```python
from build123d import *

# Parameters (mm, degrees)
BOSS_EXTRUDE1_DEPTH = 27.94
CIRPATTERN1_COUNT   = 17
SKETCH5_R           = 7.9375
SKETCH5_W           = 9.525
SKETCH5_H           = 11.576298251
CUT_EXTRUDE1_DEPTH  = 12.7
SKETCH5_2_R         = 7.9375
CUT_EXTRUDE2_DEPTH  = 70


with BuildPart() as part:
    # Sketch2 → Revolve1 (revolve)
    with BuildSketch(Plane(origin=(0, 0, 0), x_dir=(1, 0, 0), z_dir=(0, 1, 0))):
        Polygon((0, -14.35), (0, -58.593750066), (-19.05, -58.593750066), (-19.05, -45.893750066), (-21, -45.893750066), (-21, -35.1), (-20, -35.1), (-20, -28.1), (-18.8, -14.35), align=None)
    revolve(axis=Axis((0, 0, 14.35), (0, 0, 1)))

    # Sketch4 → Boss-Extrude1 (add)
    with BuildSketch(Plane.XY):
        with BuildLine():
            Line((-3.454490935, 18.479894274), (-3.774098097, 16.37058898))
            ThreePointArc((-3.774098097, 16.37058898), (-4.597538233, 16.158670805), (-5.40920169, 15.905361897))
            Line((-5.40920169, 15.905361897), (-6.791343324, 17.530477913))
            Line((-6.791343324, 17.530477913), (0, 0))
            Line((0, 0), (0, 18.8))
            ThreePointArc((0, 18.8), (-1.734645158, 18.719802514), (-3.454490935, 18.479894274))
        make_face()
    boss_extrude1 = extrude(amount=BOSS_EXTRUDE1_DEPTH)

    # CirPattern1: Boss-Extrude1 ×17 about axis
    cirpattern1_axis = Axis((0, 0, 0), (0, 0, 1))
    for i in range(1, CIRPATTERN1_COUNT):
        add(boss_extrude1.rotate(cirpattern1_axis, i * 360 / CIRPATTERN1_COUNT))

    # Sketch5 → Cut-Extrude1 (cut)
    with BuildSketch(Plane.XY.offset(58.593750066)):
        Circle(SKETCH5_R)
        with Locations((0, 19.470732312)):
            Rectangle(SKETCH5_W, SKETCH5_H)
    extrude(amount=-CUT_EXTRUDE1_DEPTH, mode=Mode.SUBTRACT)

    # Sketch5_2 → Cut-Extrude2 (cut)
    with BuildSketch(Plane.XY.offset(58.593750066)):
        Circle(SKETCH5_2_R)
    extrude(amount=-CUT_EXTRUDE2_DEPTH, mode=Mode.SUBTRACT)


solid = part.part
```
Check sheet for the modelled part. Datum: model origin and axes. Units: mm. A direction names the side the tool comes from. Coordinates: 2 decimals unless noted, no trailing zeros. Write each loop counter-clockwise with the first axis right and the second up, starting at its lowest first coordinate (ties: lowest second). Pieces come first, ordered by that corner, then holes. Notation, with made-up numbers: M -27.5,54.5 L -11.5,54.5 A21 ccw -11.5,83.5 Z; hole C 24.5,-7.5 d11. An arc over 180 degrees is marked long. Write item = value, one per line. Start each with the question number.
1. Tool access check on faces 1 (the flat face through (-4.762, 16, 52)), 2 (the flat face through (-14.419, 10.455, 7.075)), 3 (the flat face through (17.032, 5.206, 7.075)), 4 (the cylindrical face through (12.407, -11.327, 7.075)), 5 (the flat face through (2.917, -17.541, 7.075)). Record the directions out of +Z, -Z, +X, -X, +Y, -Y that give a thin tool (end or side, any length) a straight path to the whole face; none if there is none.
2. Thickness scan on probe 1 along Y at (x, z) = (0, 40); probe 2 along X at (y, z) = (0.5, 17.5); probe 3 along X at (y, z) = (-17, 9). Record the ranges inside material, lowest first.
3. Sectioned sample at D-D (z = 19). Record the cut outline in (x, y) (1 decimal).
4. Sectioned sample at C-C (z = 26). Record the cut outline in (x, y) (1 decimal).
5. Sectioned sample at A-A (y = 0). Record the cut outline in (x, z), then the cut area to 3 significant figures.
6. Mould release check, pull along X, two halves, no side actions. Record for faces 6 (the flat face through (-11.714, 13.378, 7.075)), 7 (the cylindrical face through (18.484, 3.431, 7.075)), 8 (the flat face through (-19, 8, 35.1)), 9 (the cylindrical face through (-14.29, -8.83, 7.07)): pulls with the +X half, pulls with the -X half, needs draft (parallel to the pull), parting line crosses it, or undercut.
7. Go/stop test with flat-tipped pins: pin 1 (0.8 mm diameter, centred on x = -5, y = 17.5, fed in from -Z); pin 2 (5 mm diameter, centred on y = 5, z = 42, fed in from -X); pin 3 (12.5 mm diameter, centred on x = 0, y = 0, fed in from +Z); pin 4 (5 mm diameter, centred on x = -9, z = 24, fed in from -Y). Record where each tip stops, or that it passes through.
The answers:
q1.face_1 = +Z, +Y
q1.face_2 = -Z, -X
q1.face_3 = -Z, +X
q1.face_4 = -Z
q1.face_5 = -Z, -Y
q2.probe_1 = -21 to -7.94, 7.94 to 21
q2.probe_2 = -19.07 to -7.92, 7.92 to 19.07
q2.probe_3 = -8.03 to -6.34, -3.68 to 0.63, 2.61 to 6.77
q3.outline = C 0,0 d38.4; hole C 0,0 d15.9
q4.outline = C 0,0 d39.6; hole C 0,0 d15.9
q5.outline = M -21,35.1 L -20,35.1 L -20,28.1 L -18.8,14.35 L -18.8,0 L -7.94,0 L -7.94,58.59 L -19.05,58.59 L -19.05,45.89 L -21,45.89 Z; M 7.94,0 L 16.8,0 L 16.8,14.35 L 18.8,14.35 L 20,28.1 L 20,35.1 L 21,35.1 L 21,45.89 L 19.05,45.89 L 19.05,58.59 L 7.94,58.59 Z
q5.area = 1,330 mm²
q6.face_6 = undercut
q6.face_7 = pulls with the +X half
q6.face_8 = needs draft
q6.face_9 = undercut
q7.pin_1 = 14.35
q7.pin_2 = -20.85
q7.pin_3 = through
q7.pin_4 = -18.57
